from build123d import *

# Parameters (mm, degrees)
F1_DEPTH = 370
F2_DEPTH = 400
F3_W     = 18.6485039899
F3_H     = 8
F3_W_2   = 19.9612321942
F3_R     = 3.4
F3_R_2   = 2.1
F4_DEPTH = 370
F5_R     = 2


# Not quite as in the source:
# - a pattern or mirror of a feature is missing from the dataset's text; its kind, count and spacing are read off the source's solid


with BuildPart() as f1:
    # F0 (on Front) → F1 (new body)
    with BuildSketch(Plane.XZ):
        Polygon((15, -15), (15, 15), (4, 15), (4, 13), (8.25, 13), (8.25, 9.5), (4.75, 6), (-4.75, 6), (-8.25, 9.5), (-8.25, 13), (-4, 13), (-4, 15), (-15, 15), (-15, -15), align=None)
        Polygon((4, 13), (4, 15), (-4, 15), (-4, 13), (-8.25, 13), (-8.25, 9.5), (-4.75, 6), (4.75, 6), (8.25, 9.5), (8.25, 13), align=None)
    extrude(amount=F1_DEPTH)

    # F0 (on Front) → F2 (cut)
    with BuildSketch(Plane.XZ):
        Polygon((4, 13), (4, 15), (-4, 15), (-4, 13), (-8.25, 13), (-8.25, 9.5), (-4.75, 6), (4.75, 6), (8.25, 9.5), (8.25, 13), align=None)
    f2 = extrude(amount=F2_DEPTH, mode=Mode.SUBTRACT)

    # F2_copies: F2 across plane
    add(f2.mirror(Plane(origin=(0, 0, 0), x_dir=(-1, 0, 0), z_dir=(0, 0, -1))), mode=Mode.SUBTRACT)

    # F3 (on face) → F4 (cut)
    with BuildSketch(Plane(origin=(0, 0, 0), x_dir=(-1, 0, 0), z_dir=(0, 1, 0))):
        Polygon((-6, 4.75), (-9.5, 8.25), (-13, 8.25), (-13, 4), (-13, -4), (-13, -8.25), (-9.5, -8.25), (-6, -4.75), align=None)
        with Locations((-22.3242519949, 0)):
            Rectangle(F3_W, F3_H)
        Polygon((13, 8.25), (9.5, 8.25), (6, 4.75), (6, -4.75), (9.5, -8.25), (13, -8.25), (13, -4), (13, 4), align=None)
        with Locations((22.9806160971, 0)):
            Rectangle(F3_W_2, F3_H)
        Circle(F3_R)
        with Locations((-11.6, 11.6)):
            Circle(F3_R_2)
        with Locations((-11.6, -11.6)):
            Circle(F3_R_2)
        with Locations((11.6, -11.6)):
            Circle(F3_R_2)
        with Locations((11.6, 11.6)):
            Circle(F3_R_2)
    extrude(amount=-F4_DEPTH, mode=Mode.SUBTRACT)

    # F5
    f5_edges = [f1.edges().sort_by_distance(p)[0] for p in [
        (-15, -185, 15),
        (-15, -185, -15),
        (15, -185, -15),
        (15, -185, 15),
    ]]
    fillet(f5_edges, radius=F5_R)


solid = f1.part
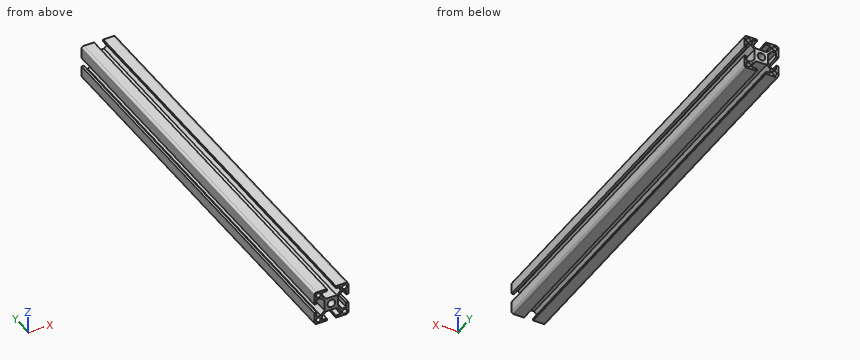
Here's how the part is built. I have some questions about the finished solid (model axes, mm). Round coordinates to 2 decimals unless told otherwise and drop trailing zeros. Write each loop counter-clockwise with the first axis right and the second up, starting at its lowest first coordinate (ties: lowest second). Pieces come first, ordered by that corner, then holes.
1. Suppose I cut it at C-C (y = -198.5). State how many separate pieces and enclosed holes the cut face has, and give its area (3 significant figures).
2. Suppose I cut it at B-B (x = 0). List the corners of the cut face in (y, z) for me.
3. Suppose I cut it at A-A (z = 0). List the corners of the cut face in (x, y) for me, and give its area (3 significant figures).
4. Will these pins go through, and if not, where does the flat tip stop? pin 1 Ø3 at (x, y) = (1.5, -55.5) entering from -Z; pin 2 Ø5 at (y, z) = (-162.5, 0) entering from +X; pin 3 Ø0.6 at (x, y) = (14.5, -182.5) entering from -Z.
5. I need wall thicknesses on L1, parallel to Z at x = -11.6, y = -275; L2, parallel to Z at x = -13.25, y = -124.5; L3, parallel to X at y = -181.5, z = 7.75. Which ranges of each line are inside material? Lowest first, please.
Answer sheet:
1. separate pieces: 1
1. enclosed holes: 5
1. area: 328 mm2
2. outline: (-370, -6) - (0, -6) - (0, -3.4) - (-370, -3.4) - close; (-370, 3.4) - (0, 3.4) - (0, 6) - (-370, 6) - close
3. outline: (-6, -370) - (-3.4, -370) - (-3.4, 0) - (-6, 0) - close; (3.4, -370) - (6, -370) - (6, 0) - (3.4, 0) - close
3. area: 1,920 mm2
4. pin 1: stops at z = -6
4. pin 2: stops at x = 6
4. pin 3: stops at z = -14.6
5. L1: z = -15 to -13.7, -9.5 to -8.25, 8.25 to 9.5, 13.7 to 15
5. L2: z = -14.98 to -12.9, -10.3 to -4, 4 to 10.3, 12.9 to 14.98
5. L3: x = -15 to -13, -9 to -6.5, 6.5 to 9, 13 to 15
